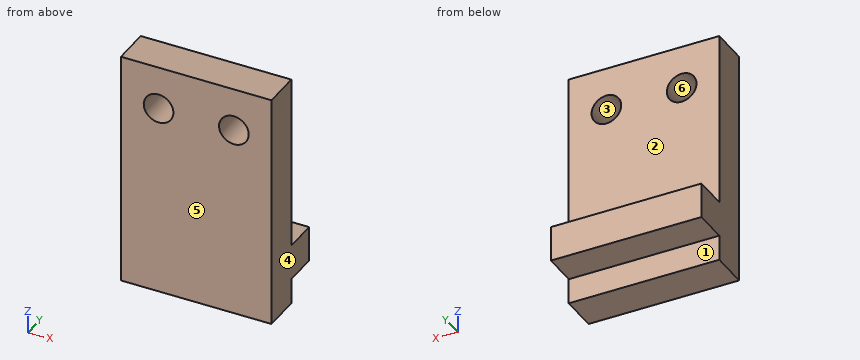
Autodesk Inventor part; units mm, degrees
ref_plane "YZ Plane" through (0, 0, 0) normal (1, 0, 0) x (0, 1, 0)
ref_plane "XZ Plane" through (0, 0, 0) normal (0, 1, 0) x (-1, 0, 0)
ref_plane "XY Plane" through (0, 0, 0) normal (0, 0, 1) x (1, 0, 0)
sketch "Sketch1" plane through (0, 0, 0) normal (0, 1, 0) x (-1, 0, 0)
  line L0 (0, 0) -> (25.4, 0)
  line L1 (25.4, 0) -> (25.4, -40.005)
  line L2 (25.4, -40.005) -> (0, -40.005)
  line L3 (0, -40.005) -> (0, 0)
  dimension "d0" = 40.005
  dimension "d1" = 25.4
extrude "Extrusion1" add sketch "Sketch1" along normal blind 6.35
sketch "Sketch2" plane through (0, 6.35, 0) normal (0, 1, 0) x (1, 0, 0)
  line L0 (-25.4, 40.005) -> (-25.4, 0)
  line L1 (0, 0) -> (0, 40.005)
  line L2 (-25.4, 35.6997) -> (0, 35.6997)
  line L3 (0, 35.6997) -> (0, 29.7053)
  line L4 (0, 29.7053) -> (-25.4, 29.7053)
  line L5 (-25.4, 29.7053) -> (-25.4, 35.6997)
  line L6 (-25.4, 32.7025) -> (0, 32.7025) construction
  line L7 (-25.4, 7.3025) -> (0, 7.3025)
  line L8 (-25.4, 0) -> (0, 0)
  line L9 (0, 40.005) -> (-25.4, 40.005)
  line L10 (-25.4, 29.7053) -> (0, 29.7053)
  line L11 (0, 29.7053) -> (0, 35.6997)
  line L12 (0, 35.6997) -> (-25.4, 35.6997)
  line L13 (-25.4, 35.6997) -> (-25.4, 29.7053)
  point P0 (-19.05, 7.3025)
  point P1 (-6.35, 7.3025)
  dimension "d4" = 5.9944
  dimension "d5" = 25.4
  dimension "d6" = 7.3025
  dimension "d7" = 40.005
  dimension "d8" = 12.7
  dimension "d9" = 25.4
  dimension "d10" = 6.35
extrude "Extrusion2" add sketch "Sketch2" along normal blind 5.715 contours L2 L1 L4 L0
hole "Hole1" at (-19.05, 6.35, -7.3025) at (-6.35, 6.35, -7.3025) direction (0, -1, 0) diameter 5 end through all
equation "\"d6\" = -0.5 * d5 + 0.5 * d7"
properties part number "slider v1"
Geometry: final body of the model. Coordinates: model frame, mm. Face numbers are marked on the shaded views. A direction names the side the tool comes from. Coordinates: 2 decimals unless noted, no trailing zeros. Order: outer loops, then holes, each group sorted by start corner. A loop starts at its lowest first (then second) coordinate and runs counter-clockwise, first axis right, second up.
Item 1: Section query D-D (z = -19). Output: boundary loops of the cut face in (x, y), then the cut area to 3 significant figures.
Answer:
outline: (-25.4, 0) - (0, 0) - (0, 6.35) - (-25.4, 6.35) - close
area: 161 mm2
Item 2: Material intervals for line 1 along Z through (x, y) = (-6.35, 2.5) (1 decimal); line 2 along X through (y, z) = (1, -7); line 3 along Y through (x, z) = (-2, -10), sorted ascending.
Answer:
line 1: z = -40 to -9.8, -4.8 to 0
line 2: x = -25.4 to -21.53, -16.57 to -8.83, -3.87 to 0
line 3: y = 0 to 6.35
Item 3: Draft query along X for the marked faces 4, 5 and 6. Return one class per face: released by +X, released by -X, zero draft, split by the parting line, or undercut.
Answer:
face 4: released by +X
face 5: zero draft
face 6: undercut
Item 4: Contact query for flat-ended pins moving along their axis: P1, Ø8, axis at x = -2.5, z = -25, coming from the +Y side; P2, Ø3, axis at y = 9.5, z = -9, coming from the -X side. Output: stop coordinate, or through.
Answer:
P1: stops at y = 6.35
P2: passes through
Item 5: Section query B-B (x = -14). Output: boundary loops of the cut face in (y, z) (3 decimals), then the cut area to 3 significant figures.
Answer:
outline: (0, -40.005) - (6.35, -40.005) - (6.35, -35.7) - (12.065, -35.7) - (12.065, -29.705) - (6.35, -29.705) - (6.35, 0) - (0, 0) - close
area: 288 mm2
Item 6: Access query for the marked faces 1, 2 and 3. Directions: +Z, -Z, +X, -X, +Y, -Y. A direction counts if a zero-diameter tool reaches every point of the face in a straight line with its end or side. Return the directions, or none.
Answer:
face 1: -Z, +X, -X, +Y
face 2: +Z, +X, -X, +Y
face 3: +Y, -Y
Item 7: Section query C-C (y = 2.5). State how many separate pieces and enclosed holes the cut face has, then the cut area to 3 significant figures.
Answer:
separate pieces: 1
enclosed holes: 2
area: 977 mm2
